CAD build for the part. Positions are in the model's coordinates, mm. Give positions to 0.01 mm unless a question says otherwise; leave off trailing zeros. Order: outer loops, then holes, each group sorted by start corner. A loop starts at its lowest first (then second) coordinate and runs counter-clockwise, first axis right, second up.
Item 1: Band-saw the part on B-B on x = 232. Count the separate pieces of the cut face and the enclosed holes in it, plus the area to 3 significant figures.
Item 2: Two-plate mould, pull along Y, no slides. Class faces 1 (the cylindrical face through (247.42, 54.38, 0.3)), 2 (the cylindrical face through (247.442, 62.198, 14.938)), 3 (the cylindrical face through (217.332, 79.715, 29.999)): released by +Y, released by -Y, zero draft, split by the parting line, or undercut.
Item 3: Wall check: L1, parallel to X at y = 76, z = 11; L2, parallel to X at y = 62.5, z = 17; L3, parallel to Y at x = 210.5, z = 22. Give the ranges that are in metal, low to high.
Item 4: Flat gauge pins, fed straight in: P1, Ø2, axis at x = 225.5, z = 20, coming from the -Y side; P2, Ø2.5, axis at x = 231.69, y = 74.94, coming from the +Z side; P3, Ø8, axis at x = 227, z = 17.5, coming from the -Y side; P4, Ø1.5, axis at x = 237, z = 10.5, coming from the -Y side. Where does each tip first touch, or does it go through?
Item 5: Band-saw the part on A-A on z = 25.5. Give the cut face in (x, y).
```python
from build123d import *

# Parameters (mm, degrees)
SKETCH_1_R               = 10.25
EXTRUDE_1_DEPTH          = 30.3
CUT_EXTRUDE_1_DEPTH      = 268.033508634
CUT_EXTRUDE_1_DEPTH_BACK = 268.033508634
SKETCH_2_R               = 1.5
FILLET_1_R               = 1


with BuildPart() as part:
    # 草图1 → 凸台-拉伸1 (new body)
    with BuildSketch(Plane.XY):
        with BuildLine():
            Line((205.951402916, 77), (205.951402916, 60))
            ThreePointArc((205.951402916, 60), (207.664953018, 51.900262342), (212.511977929, 45.188455313))
            ThreePointArc((212.511977929, 45.188455313), (214.967004798, 43.973894607), (217.693564254, 44.235023248))
            ThreePointArc((217.693564254, 44.235023248), (228.082885446, 46.993654106), (238.826448864, 47.345625871))
            ThreePointArc((238.826448864, 47.345625871), (241.077132686, 47.68338128), (242.944957082, 48.983722931))
            Line((242.944957082, 48.983722931), (252.189519734, 59.250849906))
            ThreePointArc((252.189519734, 59.250849906), (252.955973862, 61.415249594), (251.967477077, 63.487676201))
            Line((251.967477077, 63.487676201), (239.334015044, 74.86289651))
            ThreePointArc((239.334015044, 74.86289651), (233.118761907, 78.67160853), (225.951402916, 80))
            Line((225.951402916, 80), (208.951402916, 80))
            ThreePointArc((208.951402916, 80), (206.830082573, 79.121320344), (205.951402916, 77))
        make_face()
        with Locations((225.951402916, 60)):
            Circle(SKETCH_1_R, mode=Mode.SUBTRACT)
    extrude(amount=EXTRUDE_1_DEPTH)

    # 草图2 → 切除-拉伸1 (cut, two sides: drawn at the far end of the back side and taken through both)
    with BuildSketch(Plane.XY.offset(30.3).offset(-CUT_EXTRUDE_1_DEPTH_BACK)):
        with Locations((215.871834176, 48.891341485)):
            Circle(SKETCH_2_R)
        with Locations((209.951402916, 60)):
            Circle(SKETCH_2_R)
        with Locations((209.951402916, 76)):
            Circle(SKETCH_2_R)
        with Locations((231.685290109, 74.937286824)):
            Circle(SKETCH_2_R)
        with Locations((239.229232955, 52.329375962)):
            Circle(SKETCH_2_R)
        with Locations((248.547809826, 61.184227506)):
            Circle(SKETCH_2_R)
    extrude(amount=CUT_EXTRUDE_1_DEPTH + CUT_EXTRUDE_1_DEPTH_BACK, mode=Mode.SUBTRACT)

    # 圆角1
    fillet_1_edges = [part.edges().sort_by_distance(p)[0] for p in [
        (205.951402916, 68.5, 0),
        (205.951402916, 68.5, 30.3),
        (206.830082573, 79.121320344, 0),
        (206.830082573, 79.121320344, 30.3),
        (207.664953018, 51.900262342, 0),
        (207.664953018, 51.900262342, 30.3),
        (217.451402916, 80, 0),
        (214.967004798, 43.973894607, 0),
        (233.118761907, 78.67160853, 0),
        (228.082885446, 46.993654106, 0),
        (245.65074606, 69.175286355, 0),
        (241.077132686, 47.68338128, 0),
        (252.955973862, 61.415249594, 0),
        (247.567238408, 54.117286418, 0),
        (215.701402916, 60, 0),
        (217.451402916, 80, 30.3),
        (214.967004798, 43.973894607, 30.3),
        (233.118761907, 78.67160853, 30.3),
        (228.082885446, 46.993654106, 30.3),
        (245.65074606, 69.175286355, 30.3),
        (241.077132686, 47.68338128, 30.3),
        (252.955973862, 61.415249594, 30.3),
        (247.567238408, 54.117286418, 30.3),
        (215.701402916, 60, 30.3),
    ]]
    fillet(fillet_1_edges, radius=FILLET_1_R)


solid = part.part
```
The answers:
1. separate pieces: 3
1. enclosed holes: 0
1. area: 367 mm2
2. face 1: released by -Y
2. face 2: undercut
2. face 3: released by +Y
3. L1: x = 205.95 to 208.45, 211.45 to 230.63, 232.74 to 237.95
3. L2: x = 205.95 to 216.01, 235.89 to 247.83, 249.27 to 252.69
3. L3: y = 47.3 to 58.6, 61.4 to 74.6, 77.4 to 80
4. P1: stops at y = 46.32
4. P2: passes through
4. P3: stops at y = 45.96
4. P4: stops at y = 47.42
5. outline: (205.95, 60) arc R20 ccw to (212.51, 45.19) arc R5 ccw to (217.69, 44.24) arc R47.5 cw to (238.83, 47.35) arc R5 ccw to (242.94, 48.98) - (252.19, 59.25) arc R3 ccw to (251.97, 63.49) - (239.33, 74.86) arc R20 ccw to (225.95, 80) - (208.95, 80) arc R3 ccw to (205.95, 77) - close; hole circle Ø3 at (209.95, 60); hole circle Ø3 at (209.95, 76); hole circle Ø3 at (215.87, 48.89); hole circle Ø20.5 at (225.95, 60); hole circle Ø3 at (231.69, 74.94); hole circle Ø3 at (239.23, 52.33); hole circle Ø3 at (248.55, 61.18)
